from build123d import *

# Parameters (mm, degrees)
SKETCH1_W                = 130
SKETCH1_H                = 15
BOSS_EXTRUDE1_DEPTH      = 250
SKETCH2_W                = 20
SKETCH2_H                = 20
BOSS_EXTRUDE3_DEPTH      = 100
BOSS_EXTRUDE4_DEPTH      = 10
BOSS_EXTRUDE4_DEPTH_BACK = 30
SKETCH3_R                = 20
SKETCH3_R_2              = 10
SKETCH4_R                = 10
CUT_EXTRUDE1_DEPTH       = 185.407836059
FILLET1_R                = 10


with BuildPart() as part:
    # Sketch1 → Boss-Extrude1 (new body)
    with BuildSketch(Plane.XY):
        Rectangle(SKETCH1_W, SKETCH1_H)
    extrude(amount=BOSS_EXTRUDE1_DEPTH)

    # Sketch2 → Boss-Extrude3 (add)
    with BuildSketch(Plane.XZ.offset(7.5)):
        with Locations((0, 125)):
            Rectangle(SKETCH2_W, SKETCH2_H)
    extrude(amount=BOSS_EXTRUDE3_DEPTH)

    # Sketch3 → Boss-Extrude4 (add, two sides: drawn at the far end of the back side and taken through both)
    with BuildSketch(Plane.XY.offset(135).offset(-BOSS_EXTRUDE4_DEPTH_BACK)):
        with Locations((0, -77.5)):
            Circle(SKETCH3_R)
        with Locations((0, -77.5)):
            Circle(SKETCH3_R_2, mode=Mode.SUBTRACT)
    extrude(amount=BOSS_EXTRUDE4_DEPTH + BOSS_EXTRUDE4_DEPTH_BACK)

    # Sketch4 → Cut-Extrude1 (cut, through all)
    with BuildSketch(Plane.XY.offset(135)):
        with Locations((0, -77.5)):
            Circle(SKETCH4_R)
    extrude(amount=-CUT_EXTRUDE1_DEPTH, mode=Mode.SUBTRACT)

    # Fillet1
    fillet1_edges = [part.edges().sort_by_distance(p)[0] for p in [
        (10, -107.5, 125),
        (0, -107.5, 135),
        (-10, -107.5, 125),
        (0, -107.5, 115),
    ]]
    fillet(fillet1_edges, radius=FILLET1_R - 0.0001)  # a hair under: the kernel refuses the full size


solid = part.part
Design review of the part built by this model. Coordinates are the model's own, in mm. A direction names the side the tool comes from. Give positions to 0.01 mm unless a question says otherwise; leave off trailing zeros. Loops run counter-clockwise (first coordinate to the right, second up) from the corner with the lowest first, then second, coordinate; pieces in that order, holes last. Notation, with made-up numbers: M 39,84 L 98,84 A11 ccw 98,88 Z; hole C 34.25,-36.5 d5. An arc over 180 degrees is marked long. Answer as a JSON object with one key per item and string values.
Item 1: For P1, Ø10, axis at x = 0, y = -25.5, coming from the +Z side; P2, Ø2, axis at x = 0.5, y = -96.5, coming from the +Z side; P3, Ø16, axis at y = -41.5, z = 126.5, coming from the +X side, all flat-tipped, find the tip position at first contact; note any pin that passes through.
Output values:
{"P1": "stops at z = 135", "P2": "stops at z = 145", "P3": "stops at x = 10"}
Item 2: We need section B-B (y = -77.5). State the section outline as (x, z) points.
Output values:
{"outline": "M -20,105 L -10,105 L -10,145 L -20,145 Z; M 10,105 L 20,105 L 20,145 L 10,145 Z"}
Item 3: We need section C-C (x = 6). State the section outline as (y, z) points.
Output values:
{"outline": "M -105.5,119 A10 ccw -97.5,115 L -96.58,115 L -96.58,105 L -85.5,105 L -85.5,145 L -96.58,145 L -96.58,135 L -97.5,135 A10 ccw -105.5,131 Z; M -69.5,105 L -58.42,105 L -58.42,115 L -7.5,115 L -7.5,0 L 7.5,0 L 7.5,250 L -7.5,250 L -7.5,135 L -58.42,135 L -58.42,145 L -69.5,145 Z"}
Item 4: Wall thickness on line 1 along Y through (x, z) = (0, 124); line 2 along Y through (x, z) = (0, 125.5); line 3 along X through (y, z) = (-77, 121): over which ranges is each line inside the solid? List them lowest first.
Output values:
{"line 1": "y = -107.45 to -87.5, -67.5 to 7.5", "line 2": "y = -107.49 to -87.5, -67.5 to 7.5", "line 3": "x = -19.99 to -9.99, 9.99 to 19.99"}
Item 5: We need section A-A (x = -16). State the section outline as (y, z) points, and give its area (3 significant figures).
Output values:
{"outline": "M -89.5,105 L -65.5,105 L -65.5,145 L -89.5,145 Z; M -7.5,0 L 7.5,0 L 7.5,250 L -7.5,250 Z", "area": "4,710 mm2"}
Item 6: Machinability: for faces 1 (the face through (4, -68, 105)), 2 (the face through (-10, -33, 125)), 3 (the face through (8.128, -103.326, 125.14)), 4 (the face through (10, -33, 125)), which of the approach directions +Z, -Z, +X, -X, +Y, -Y give a long, thin tool a straight path to every point of the face, cutting with its end or side? Answer none if there is none.
Output values:
{"face 1": "-Z, +X, -X, -Y", "face 2": "+Z, -Z, -X", "face 3": "+Z, -Z, +X, -Y", "face 4": "+Z, -Z, +X"}
Item 7: We need section D-D (z = 166). State the section outline as (x, y) points.
Output values:
{"outline": "M -65,-7.5 L 65,-7.5 L 65,7.5 L -65,7.5 Z"}
Item 8: Mouldability with a two-part tool opening along X and no side actions: class faces 5 (the face through (-8.25, -103.15, 125.14)), 6 (the face through (4, -68, 145)), 7 (the face through (5.38, -69.07, 124.72)) as pulls with the +X half, pulls with the -X half, needs draft (parallel to the pull), parting line crosses it, or undercut.
Output values:
{"face 5": "pulls with the -X half", "face 6": "needs draft", "face 7": "undercut"}
